Geometry: final body of the model. Coordinates: model frame, mm. A direction names the side the tool comes from. Coordinates: 2 decimals unless noted, no trailing zeros. Order: outer loops, then holes, each group sorted by start corner. A loop starts at its lowest first (then second) coordinate and runs counter-clockwise, first axis right, second up. Notation, with made-up numbers: (62.5, 0.5) - (88.5, 0.5) arc R21 cw to (88.5, 37.5) - close; hole circle Ø9 at (-7.5, -14.75). An arc over 180 degrees is marked (long way). Use a Markdown table: item, result. Add a question column.
Autodesk Inventor part; units mm, degrees
ref_plane "YZ Plane" through (0, 0, 0) normal (1, 0, 0) x (0, 1, 0)
ref_plane "XZ Plane" through (0, 0, 0) normal (0, 1, 0) x (-1, 0, 0)
ref_plane "XY Plane" through (0, 0, 0) normal (0, 0, 1) x (1, 0, 0)
sketch "Skizze1" plane through (0, 0, 0) normal (0, 1, 0) x (-1, 0, 0)
  line L0 (0, 0) -> (48, 0)
  line L1 (48, 0) -> (48, -63) construction
  line L2 (48, -63) -> (0, -63)
  line L3 (0, -63) -> (0, 0)
  arc A0 (44, -63) -> (44, 0) centre (-78.0312, -31.5) ccw
  line L4 (44, 0) -> (44, -63) construction
  line L5 (44, 0) -> (107, 0) construction
  dimension "d0" = 48
  dimension "d1" = 63
  dimension "d2" = 90
extrude "Extrusion1" add sketch "Skizze1" along normal blind 1
sketch "Skizze2" plane through (0, 1, 0) normal (0, 1, 0) x (1, 0, 0)
  line L0 (-44, 0) -> (0, 0)
  line L1 (0, 0) -> (0, 63)
  line L2 (0, 63) -> (-44, 63)
  arc A0 (-44, 63) -> (-44, 0) centre (78.0312, 31.5) ccw
  circle A1 centre (-42, 3.5) radius 1
  circle A2 centre (-2.5, 1.5) radius 1
  circle A3 centre (-44, 22.5) radius 1
  circle A4 centre (-42, 60.5) radius 1
  circle A5 centre (-3, 58.5) radius 1
  circle A6 centre (-3, 39.5) radius 1
  line L3 (-38, 8.5) -> (-28, 8.5)
  line L4 (-28, 8.5) -> (-28, 18.5)
  line L5 (-28, 18.5) -> (-38, 18.5)
  line L6 (-38, 18.5) -> (-38, 8.5)
  point P0 (0, 0)
  dimension "d5" = 2
  dimension "d6" = 3.5
  dimension "d7" = 2
  dimension "d8" = 2
  dimension "d9" = 2
  dimension "d10" = 39.5
  dimension "d11" = 2
  dimension "d12" = 2
  dimension "d13" = 19
  dimension "d14" = 2
  dimension "d15" = 57
  dimension "d16" = 2
  dimension "d17" = 2
  dimension "d18" = 39
  dimension "d19" = 2
  dimension "d20" = 19
  dimension "d21" = 10
  dimension "d22" = 10
  dimension "d23" = 5
  dimension "d24" = 4
extrude "Extrusion2" cut sketch "Skizze2" against normal through all contours A1 | A2 | A3 | A4 | A5 | A6 | L6 L5 L4 L3
sketch "Skizze3" plane through (0, 1, 0) normal (0, 1, 0) x (1, 0, 0)
  circle A0 centre (-3, 39.5) radius 1
  circle A1 centre (-42, 60.5) radius 1
  circle A2 centre (-2.5, 1.5) radius 1
  circle A3 centre (-42, 3.5) radius 1
  circle A4 centre (-44, 22.5) radius 1
  circle A5 centre (-3, 58.5) radius 1
  line L0 (-28, 18.5) -> (-28, 8.5)
  line L1 (-28, 8.5) -> (-38, 8.5)
  line L2 (-38, 8.5) -> (-38, 18.5)
  line L3 (-38, 18.5) -> (-28, 18.5)
  line L4 (-44, 0) -> (0, 0)
  line L5 (0, 0) -> (0, 63)
  line L6 (0, 63) -> (-44, 63)
  arc A6 (-44, 63) -> (-44, 0) centre (78.0312, 31.5) ccw
  line L7 (-28, 8.5) -> (-38, 8.5)
  line L8 (-38, 8.5) -> (-28, 8.5)
  line L9 (-28, 8.5) -> (-28, 18.5)
  line L10 (-28, 18.5) -> (-38, 18.5)
  line L11 (-38, 18.5) -> (-38, 8.5)
  line L12 (-38, 0) -> (-7, 0)
  line L13 (-7, 0) -> (-7, 41)
  line L14 (-7, 41) -> (-38, 41)
  line L15 (-38, 41) -> (-38, 0)
  line L16 (-7, 41) -> (-34, 41)
  line L17 (-34, 41) -> (-34, 55)
  line L18 (-34, 55) -> (-7, 55)
  line L19 (-7, 55) -> (-7, 41)
  point P0 (0, 0)
  dimension "d27" = 31
  dimension "d28" = 41
  dimension "d31" = 27
  dimension "d32" = 8
extrude "Extrusion3" add sketch "Skizze3" along normal blind 1 contours L3 L15 L14 L13 L4 L1 L0 | L0 L1 L2 L3 | L17 L18 L19 L14
sketch "Skizze4" plane through (0, 2, 0) normal (0, 1, 0) x (1, 0, 0)
  line L0 (-38, 18.5) -> (-28, 18.5)
  line L1 (-28, 18.5) -> (-28, 8.5)
  line L2 (-28, 8.5) -> (-38, 8.5)
  line L3 (-38, 8.5) -> (-38, 18.5)
  point P0 (0, 0)
extrude "Extrusion4" add sketch "Skizze4" along normal blind 4
properties part number "00_Backplate"
1) Section query A-A (x = -42). Return the cut outline in (y, z).
2) Section query C-C (x = -17.5). Return the cut outline in (y, z), and give its area (3 significant figures).
3) Draft query along X for faces 4 (the flat face through (-28, 4, -14)), 5 (the cylindrical face through (-2.46, 0.51, -59.34)), 6 (the flat face through (-33, 4, -8.5)). Return one class per face: released by +X, released by -X, zero draft, split by the parting line, or undercut.
4) First-contact query: pin 1 (6 mm diameter, centred on x = -13, z = -46, fed in from +Y); pin 2 (2.5 mm diameter, centred on y = 3, z = -11.5, fed in from -X); pin 3 (2.5 mm diameter, centred on x = -3, z = -58.5, fed in from +Y); pin 4 (3 mm diameter, centred on x = -2.5, z = -1.5, fed in from -Y). Flat tips, straight axial feed; report the tip coordinate or a pass-through.
5) Section query D-D (z = -39.5). Return the cut outline in (x, y).
6) Section query B-B (z = -60.5). Return the cut outline in (x, y), and give its area (3 significant figures).
7) Access query for faces 1 (the flat face through (-38, 2, -16)), 2 (the flat face through (-33, 4, -18.5)), 3 (the flat face through (-33, 1, -14)). Directions: +Z, -Z, +X, -X, +Y, -Y. A direction counts if a zero-diameter tool reaches every point of the face in a straight line with its end or side. Return the directions, or none.
8) Line query: line 1 (Z direction, x = -42, y = 0.35); line 2 (Z direction, x = -3, y = 0.5); line 3 (Y direction, x = -34, z = -28). Output: solid intervals per line, ascending. Write a range as from..to.
From the geometry:
| question | item | result |
|---|---|---|
| 1 | outline | (0, -63) - (1, -63) - (1, -61.5) - (0, -61.5) - close; (0, -59.5) - (1, -59.5) - (1, -4.5) - (0, -4.5) - close; (0, -2.5) - (1, -2.5) - (1, 0) - (0, 0) - close |
| 2 | outline | (0, -63) - (1, -63) - (1, -55) - (2, -55) - (2, 0) - (0, 0) - close |
| 2 | area | 118 mm^2 |
| 3 | face 4 | released by +X |
| 3 | face 5 | undercut |
| 3 | face 6 | zero draft |
| 4 | pin 1 | stops at y = 2 |
| 4 | pin 2 | stops at x = -38 |
| 4 | pin 3 | stops at y = 1 |
| 4 | pin 4 | stops at y = 0 |
| 5 | outline | (-47.75, 0) - (-4, 0) - (-4, 1) - (-7, 1) - (-7, 2) - (-38, 2) - (-38, 1) - (-47.75, 1) - close; (-2, 0) - (0, 0) - (0, 1) - (-2, 1) - close |
| 6 | outline | (-44.62, 0) - (-43, 0) - (-43, 1) - (-44.62, 1) - close; (-41, 0) - (0, 0) - (0, 1) - (-41, 1) - close |
| 6 | area | 42.6 mm^2 |
| 7 | face 1 | +Z, -Z, -X, +Y |
| 7 | face 2 | -Z, +X, -X, +Y |
| 7 | face 3 | -Y |
| 8 | line 1 | z = -63..-61.5, -59.5..-4.5, -2.5..0 |
| 8 | line 2 | z = -63..-59.5, -57.5..-40.5, -38.5..-2.37, -0.63..0 |
| 8 | line 3 | y = 0..2 |
